The drawing under review shows one solid part. Ordinate dimensions are in mm from its lowest x, y, z. A direction names the side the tool comes from. Round coordinates to 2 decimals unless told otherwise and drop trailing zeros. Loops run counter-clockwise (first coordinate to the right, second up) from the corner with the lowest first, then second, coordinate; pieces in that order, holes last. Notation, with made-up numbers: M 17,42.25 L 56,42.25 A30 ccw 56,81.25 Z; hole C 80,4.25 d11. An arc over 180 degrees is marked long. Use a Markdown table: item, result.
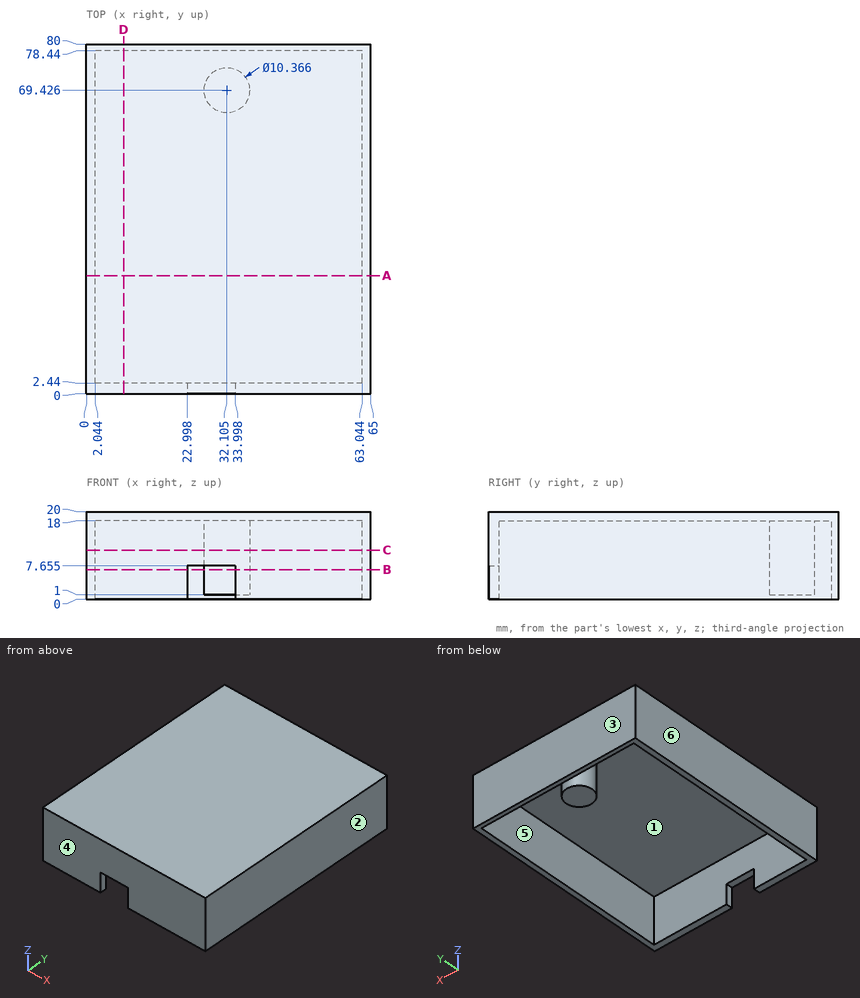
1. The part is to be moulded in two halves that separate along Y. For the marked faces 1, 2, 3 and 4, say which applies: pulls with the +Y half, pulls with the -Y half, needs draft (parallel to the pull), parting line crosses it, or undercut.
Check values:
| item | result |
|---|---|
| face 1 | undercut |
| face 2 | needs draft |
| face 3 | pulls with the +Y half |
| face 4 | pulls with the -Y half |
2. Machinability: for the marked faces 5 and 6, which of the approach directions +Z, -Z, +X, -X, +Y, -Y give a long, thin tool a straight path to every point of the face, cutting with its end or side? Answer none if there is none.
Check values:
| item | result |
|---|---|
| face 5 | -Z |
| face 6 | +Z, -Z, -X, +Y, -Y |
3. Take a section at B-B on z = 6.75. Give the boundary of the cut face in (x, y) (1 decimal).
Check values:
| item | result |
|---|---|
| outline | M 0,0 L 23,0 L 23,2.4 L 2,2.4 L 2,78.4 L 63,78.4 L 63,2.4 L 34,2.4 L 34,0 L 65,0 L 65,80 L 0,80 Z; C 32.1,69.4 d10.4 |
4. Wall thickness on line 1 along Y through (x, z) = (6, 15.5); line 2 along Y through (x, z) = (32, 10.5) (1 decimal); line 3 along X through (y, z) = (62, 1): over which ranges is each line inside the solid? List them lowest first. Write a range as from..to.
Check values:
| item | result |
|---|---|
| line 1 | y = 0..2.44, 78.44..80 |
| line 2 | y = 0..2.4, 64.2..74.6, 78.4..80 |
| line 3 | x = 0..2.04, 63.04..65 |
5. Take a section at D-D on x = 8.5. Give the boundary of the cut face in (y, z), and give its area (3 significant figures).
Check values:
| item | result |
|---|---|
| outline | M 0,0 L 2.44,0 L 2.44,18 L 78.44,18 L 78.44,0 L 80,0 L 80,20 L 0,20 Z |
| area | 232 mm² |
6. Take a section at C-C on z = 11.25. Give the boundary of the cut face in (x, y) (1 decimal).
Check values:
| item | result |
|---|---|
| outline | M 0,0 L 65,0 L 65,80 L 0,80 Z; C 32.1,69.4 d10.4; hole M 2,2.4 L 63,2.4 L 63,78.4 L 2,78.4 Z |
7. Take a section at A-A on y = 27. Give the boundary of the cut face in (x, z).
Check values:
| item | result |
|---|---|
| outline | M 0,0 L 2.04,0 L 2.04,18 L 63.04,18 L 63.04,0 L 65,0 L 65,20 L 0,20 Z |
8. Insertion check: pin 1 (5.5 mm diameter, centred on x = 27.5, z = 6.5, fed in from -Y); pin 2 (2 mm diameter, centred on x = 31.5, y = 29, fed in from -Z); pin 3 (11.5 mm diameter, centred on x = 32, y = 71.5, fed in from -Z); pin 4 (1.2 mm diameter, centred on x = 28.5, y = 1, fed in from -Z) (1 decimal). Each pin has a flat end and moves straight along its axis. Give the tip position at first contact, or say it passes through.
Check values:
| item | result |
|---|---|
| pin 1 | stops at y = 0 |
| pin 2 | stops at z = 18 |
| pin 3 | stops at z = 1 |
| pin 4 | stops at z = 7.7 |
